Check sheet for the modelled part. Datum: model origin and axes. Units: mm. A direction names the side the tool comes from. Round coordinates to 2 decimals unless told otherwise and drop trailing zeros. Write each loop counter-clockwise with the first axis right and the second up, starting at its lowest first coordinate (ties: lowest second). Pieces come first, ordered by that corner, then holes.
Item 1: Cross-section at D-D on y = -27.5. Enter the section's corners in (x, z), plus the area to 3 significant figures.
Item 2: Tool access check on faces 1 (the cylindrical face through (22.155, 25.021, -3.451)), 2 (the cylindrical face through (-63, 30, 1)), 3 (the flat face through (31, 1, -1.5)). Record the directions out of +Z, -Z, +X, -X, +Y, -Y that give a thin tool (end or side, any length) a straight path to the whole face; none if there is none.
Item 3: Cross-section at A-A on z = -4.5. Enter the section's corners in (x, y).
Item 4: Release check for a two-part mould opening along Y. For faces 4 (the cylindrical face through (62.306, 28.765, 1.014)), 5 (the flat face through (31, 17, -1.5)), 6 (the cylindrical face through (64, 29, 1)), 7 (the cylindrical face through (33.198, 8.775, -0.74)) record: +Y half, -Y half, draft (parallel to the pull), parting line (faces both ways), or undercut.
Item 5: Go/stop test with flat-tipped pins: pin 1 Ø11 at (x, y) = (47, -3) entering from -Z; pin 2 Ø2 at (x, y) = (2, -12.5) entering from -Z. Record where each tip stops, or that it passes through.
Item 6: Cross-section at C-C on y = 5.5. Enter the section's corners in (x, z).
Item 7: Cross-section at B-B on x = -15.5. Enter the section's corners in (y, z), plus the area to 3 significant figures.
Item 8: Material ranges on line 1 (Y direction, x = 31, z = -0.95); line 2 (Y direction, x = 21, z = -3.75); line 3 (X direction, y = -10, z = -1), recorded low to high.
from build123d import *

# Parameters (mm, degrees)
SKETCH005_R           = 1.25
EXTRUDE004_DEPTH      = 8
SKETCH006_R           = 1.5
EXTRUDE005_DEPTH      = 2
EXTRUDE005_DEPTH_BACK = 1
SKETCH001_R           = 3.5
SKETCH001_W           = 65
SKETCH001_H           = 14
SKETCH001_W_2         = 9
SKETCH001_H_2         = 4.5
EXTRUDE003_DEPTH      = 2
SKETCH003_R           = 3.5
EXTRUDE001_DEPTH      = 7
SKETCH004_R           = 4.7625
EXTRUDE002_DEPTH      = 1.5
SKETCH007_W           = 27
SKETCH007_H           = 11
SKETCH007_W_2         = 23
SKETCH007_H_2         = 7
SKETCH007_R           = 0.9
EXTRUDE006_DEPTH      = 2
EXTRUDE_DEPTH         = 2
CHAMFER_SIZE          = 1


with BuildPart() as extrude004:
    # Sketch005 → Extrude004 (new body)
    with BuildSketch(Plane.XY):
        with Locations((-54, 25.5)):
            Circle(SKETCH005_R)
        with Locations((21, 25.5)):
            Circle(SKETCH005_R)
        with Locations((-54, -5.5)):
            Circle(SKETCH005_R)
        with Locations((21, -5.5)):
            Circle(SKETCH005_R)
    extrude(amount=-EXTRUDE004_DEPTH)


with BuildPart() as extrude005:
    # Sketch006 → Extrude005 (new body, two sides)
    with BuildSketch(Plane.XY) as extrude005_sk:
        with Locations((-61.5, 27.5)):
            Circle(SKETCH006_R)
        with Locations((61.5, 27.5)):
            Circle(SKETCH006_R)
        with Locations((-61.5, -27.5)):
            Circle(SKETCH006_R)
        with Locations((61.5, -27.5)):
            Circle(SKETCH006_R)
    extrude(amount=EXTRUDE005_DEPTH)
    extrude(extrude005_sk.sketch, amount=-EXTRUDE005_DEPTH_BACK)


with BuildPart() as fusion001:
    # Sketch001 → Extrude003 (new body, symmetric)
    with BuildSketch(Plane.XY):
        with Locations((31, 13)):
            Circle(SKETCH001_R)
        with Locations((47, 13)):
            Circle(SKETCH001_R)
        with Locations((31, -3)):
            Circle(SKETCH001_R)
        with Locations((47, -3)):
            Circle(SKETCH001_R)
        with Locations((31, -19)):
            Circle(SKETCH001_R)
        with Locations((47, -19)):
            Circle(SKETCH001_R)
        with Locations((-16.5, 10)):
            Rectangle(SKETCH001_W, SKETCH001_H)
        with Locations((-44.5, -12.5)):
            Rectangle(SKETCH001_W_2, SKETCH001_H_2)
        with Locations((11.5, -12.5)):
            Rectangle(SKETCH001_W_2, SKETCH001_H_2)
    extrude(amount=EXTRUDE003_DEPTH, both=True)

    # Fusion001: union Extrude004, Extrude005
    add(extrude004.part)
    add(extrude005.part)


with BuildPart() as extrude001:
    # Sketch003 → Extrude001 (new body)
    with BuildSketch(Plane.XY):
        with Locations((-54, 25.5)):
            Circle(SKETCH003_R)
        with Locations((21, 25.5)):
            Circle(SKETCH003_R)
        with Locations((-54, -5.5)):
            Circle(SKETCH003_R)
        with Locations((21, -5.5)):
            Circle(SKETCH003_R)
    extrude(amount=-EXTRUDE001_DEPTH)


with BuildPart() as extrude002:
    # Sketch004 → Extrude002 (new body)
    with BuildSketch(Plane.XY):
        with Locations((31, 13)):
            Circle(SKETCH004_R)
        with Locations((47, 13)):
            Circle(SKETCH004_R)
        with Locations((31, -3)):
            Circle(SKETCH004_R)
        with Locations((47, -3)):
            Circle(SKETCH004_R)
        with Locations((31, -19)):
            Circle(SKETCH004_R)
        with Locations((47, -19)):
            Circle(SKETCH004_R)
    extrude(amount=-EXTRUDE002_DEPTH)


with BuildPart() as extrude006:
    # Sketch007 → Extrude006 (new body)
    with BuildSketch(Plane.XY):
        with Locations((-44.5, -12.5)):
            Rectangle(SKETCH007_W, SKETCH007_H)
        with Locations((-44.5, -12.5)):
            Rectangle(SKETCH007_W_2, SKETCH007_H_2, mode=Mode.SUBTRACT)
        with Locations((11.5, -12.5)):
            Rectangle(SKETCH007_W, SKETCH007_H)
        with Locations((11.5, -12.5)):
            Rectangle(SKETCH007_W_2, SKETCH007_H_2, mode=Mode.SUBTRACT)
        with Locations((-54, -12.5)):
            Circle(SKETCH007_R)
        with Locations((-35, -12.5)):
            Circle(SKETCH007_R)
        with Locations((2, -12.5)):
            Circle(SKETCH007_R)
        with Locations((21, -12.5)):
            Circle(SKETCH007_R)
    extrude(amount=-EXTRUDE006_DEPTH)


with BuildPart() as chamfer_body:
    # Sketch → Extrude (new body)
    with BuildSketch(Plane.XY):
        with BuildLine():
            ThreePointArc((-60, 31), (-63.535534, 29.535534), (-65, 26))
            Line((-65, -26), (-65, 26))
            ThreePointArc((-65, -26), (-63.535534, -29.535534), (-60, -31))
            Line((60, -31), (-60, -31))
            ThreePointArc((60, -31), (63.535534, -29.535534), (65, -26))
            Line((65, 26), (65, -26))
            ThreePointArc((65, 26), (63.535534, 29.535534), (60, 31))
            Line((-60, 31), (60, 31))
        make_face()
    extrude(amount=EXTRUDE_DEPTH)

    # Fusion: union Extrude001, Extrude002, Extrude006
    add(extrude001.part)
    add(extrude002.part)
    add(extrude006.part)

    # Cut: cut Fusion001
    add(fusion001.part, mode=Mode.SUBTRACT)

    # Chamfer
    chamfer_edges = [chamfer_body.edges().sort_by_distance(p)[0] for p in [
        (-49, -12.5, 2),
        (-44.5, -14.75, 2),
        (-40, -12.5, 2),
        (-44.5, -10.25, 2),
        (7, -12.5, 2),
        (11.5, -14.75, 2),
        (16, -12.5, 2),
        (11.5, -10.25, 2),
        (-49, 10, 2),
        (-16.5, 3, 2),
        (16, 10, 2),
        (-16.5, 17, 2),
    ]]
    chamfer(chamfer_edges, length=CHAMFER_SIZE)


solid = chamfer_body.part
Response values:
1. outline: (-64.77, 0) - (-63, 0) - (-63, 2) - (-64.77, 2) - close; (-60, 0) - (60, 0) - (60, 2) - (-60, 2) - close; (63, 0) - (64.77, 0) - (64.77, 2) - (63, 2) - close
1. area: 247 mm2
2. face 1: -Z
2. face 2: +Z, -Z, -X, +Y
2. face 3: -Z, +X, +Y, -Y
3. outline: circle Ø7 at (-54, -5.5); circle Ø7 at (-54, 25.5); circle Ø7 at (21, -5.5); circle Ø7 at (21, 25.5); hole circle Ø2.5 at (-54, -5.5); hole circle Ø2.5 at (-54, 25.5); hole circle Ø2.5 at (21, -5.5); hole circle Ø2.5 at (21, 25.5)
4. face 4: undercut
4. face 5: draft
4. face 6: +Y half
4. face 7: undercut
5. pin 1: stops at z = -1.5
5. pin 2: stops at z = -2
6. outline: (-65, 0) - (-49, 0) - (-49, 1) - (-50, 2) - (-65, 2) - close; (16, 0) - (65, 0) - (65, 2) - (17, 2) - (16, 1) - close
7. outline: (-31, 0) - (3, 0) - (3, 1) - (2, 2) - (-31, 2) - close; (17, 0) - (31, 0) - (31, 2) - (18, 2) - (17, 1) - close
7. area: 95.0 mm2
8. line 1: y = -23.76 to -22.5, -15.5 to -14.24, -7.76 to -6.5, 0.5 to 1.76, 8.24 to 9.5, 16.5 to 17.76
8. line 2: y = -9 to -6.75, -4.25 to -2, 22 to 24.25, 26.75 to 29
8. line 3: x = -58 to -56, -33 to -31, -2 to 0, 23 to 25
